from build123d import *

# Parameters (mm, degrees)
F0_R     = 4
F1_DEPTH = 15
F3_DEPTH = 6.5


with BuildPart() as f1:
    # F0 (on Top) → F1 (new body)
    with BuildSketch(Plane.XY):
        Circle(F0_R)
    extrude(amount=-F1_DEPTH)

    # F2 (on face) → F3 (join)
    with BuildSketch(Plane.XY):
        Polygon((7, 3.984384), (0, 8.025836), (-7, 3.984384), (-7, -4.098519), (0, -8.139971), (7, -4.098519), align=None)
    extrude(amount=F3_DEPTH)

    # F6: sweep along a path in F5
    with BuildLine(Plane.XY.offset(6.5)) as f6_path:
        CenterArc((0, 0), 8.139971, 0, 360)
    # F4 (on Right) → F6 (sweep, cut)
    with BuildSketch(Plane.YZ):
        Polygon((-8.139971, 5.7), (-6.739971, 6.5), (-8.139971, 6.5), align=None)
    sweep(path=f6_path.line, mode=Mode.SUBTRACT)


solid = f1.part
For this review, take the finished solid that the model builds, in its own axes (mm). A direction names the side the tool comes from. Coordinates: 2 decimals unless noted, no trailing zeros. Loops run counter-clockwise (first coordinate to the right, second up) from the corner with the lowest first, then second, coordinate; pieces in that order, holes last. Notation, with made-up numbers: (37.25, 74) -> (65.25, 74) arc R24 ccw to (65.25, 88) -> close; hole circle Ø1 at (1, 72). An arc over 180 degrees is marked (long way). Write each question's results on one line, items separated by ' | '.
Q1. Machinability: for faces 1 (the flat face through (-3, -4, 0)), 2 (the flat face through (-7, 0, 3)), which of the approach directions +Z, -Z, +X, -X, +Y, -Y give a long, thin tool a straight path to every point of the face, cutting with its end or side? Answer none if there is none.
Taken from the geometry:
face 1: -Z | face 2: +Z, -Z, -X, +Y, -Y
Q2. To check wall thickness, follow line 1 along Z through (x, y) = (-1.5, 6.5); line 2 along Z through (x, y) = (-0.25, 7); line 3 along Y through (x, z) = (-6, 5.5). State the ranges of each line that lie inside material, in increasing order. Write a range as [from, to].
Taken from the geometry:
line 1: [0, 6.5] | line 2: [0, 6.35] | line 3: [-4.68, 4.56]
Q3. For pin 1 Ø1.5 at (x, z) = (-3.5, 4) entering from -Y; pin 2 Ø3 at (x, y) = (4, -6.5) entering from -Z, all flat-tipped, find the tip position at first contact; note any pin that passes through.
Taken from the geometry:
pin 1: y = -6.55 | pin 2: z = 0
Q4. Add section B-B, the plane z = 5. State the section outline as (x, y) points.
Taken from the geometry:
outline: (-7, -4.1) -> (0, -8.14) -> (7, -4.1) -> (7, 3.98) -> (0, 8.03) -> (-7, 3.98) -> close
Q5. Add section C-C, the plane z = -10. State the section outline as (x, y) points, then the cut area to 3 significant figures.
Taken from the geometry:
outline: circle Ø8 at (0, 0) | area: 50.3 mm²
Q6. Add section A-A, the plane y = 0. State the section outline as (x, z) points.
Taken from the geometry:
outline: (-7, 0) -> (-4, 0) -> (-4, -15) -> (4, -15) -> (4, 0) -> (7, 0) -> (7, 6.35) -> (6.74, 6.5) -> (-6.74, 6.5) -> (-7, 6.35) -> close
